Source: CAD feature listing. Evaluate the final solid. Frame: model axes, mm. Face numbers are marked on the shaded views. A direction names the side the tool comes from. Coordinates: 2 decimals unless noted, no trailing zeros. Write each loop counter-clockwise with the first axis right and the second up, starting at its lowest first coordinate (ties: lowest second). Pieces come first, ordered by that corner, then holes. Notation, with made-up numbers: (-29, 18.5) -> (-18, 18.5) arc R8 cw to (-18, 31.5) -> close; hole circle Ø6 at (73.5, -20). An arc over 180 degrees is marked (long way). One line per item, written item: value. Start each with the question number.
1. Line query: line 1 (X direction, y = 5.2, z = 0); line 2 (X direction, y = 3.35, z = 0); line 3 (Y direction, x = 10.5, z = 0). Output: solid intervals per line, ascending.
2. Section query C-C, the plane x = 15. Output: boundary loops of the cut face in (y, z), and give its area (3 significant figures).
3. Section query B-B, the plane x = 10.25. Output: boundary loops of the cut face in (y, z), and give its area (3 significant figures).
4. Mould query, pull axis Y, two halves, no side actions, for the marked faces 1, 2, 3 and 4. Classes: released by +Y, released by -Y, zero draft, split by the parting line, or undercut.
5. Access query for the marked faces 5, 6, 7, 8 and 9. Directions: +Z, -Z, +X, -X, +Y, -Y. A direction counts if a zero-diameter tool reaches every point of the face in a straight line with its end or side. Return the directions, or none.
6. Section query A-A, the plane y = 3. Output: boundary loops of the cut face in (x, z).
7. First-contact query: P1, Ø3, axis at x = 4.5, y = -1.5, coming from the -Z side; P2, Ø3, axis at x = 5, y = 2.5, coming from the +Z side; P3, Ø5, axis at x = 15, z = 0, coming from the +Y side; P4, Ø3.5, axis at y = 0, z = 0, coming from the -X side. Flat tips, straight axial feed; report the tip coordinate or a pass-through.
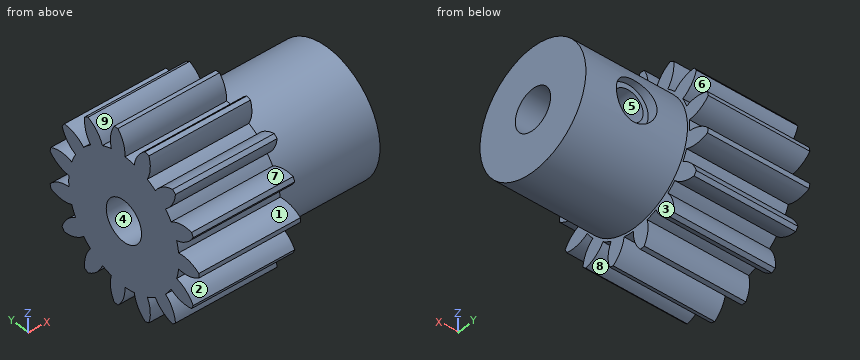
from build123d import *

# Parameters (mm, degrees)
STOCK_GEAR_1M_15T_D4_START_1_OUTLINE_R = 2
STOCK_GEAR_1M_15T_D4_START_1_DEPTH     = 10
SKETCH1_R                              = 6
SKETCH1_R_2                            = 2
BOSS_EXTRUDE1_DEPTH                    = 10
SKETCH2_R                              = 1.5
CUT_EXTRUDE2_DEPTH                     = 6
SKETCH2_3_R                            = 2
CUT_EXTRUDE3_DEPTH                     = 1


# Read off the part's stored shape, not the designer's step: Stock-Gear 1M 15T D4 Start-1
with BuildPart() as part:
    # Stock-Gear 1M 15T D4 Start-1 outline → Stock-Gear 1M 15T D4 Start-1 (new body)
    with BuildSketch(Plane.YZ):
        with BuildLine():
            ThreePointArc((1.106368468, 8.427689411), (0.888491938, 8.453436111), (0.670023493, 8.473551116))
            ThreePointArc((0.670023493, 8.473551116), (0.04560728, 7.441942771), (-0.122166634, 6.24780572))
            ThreePointArc((-0.122166634, 6.24780572), (-0.653198367, 6.214767324), (-1.179494851, 6.136676046))
            ThreePointArc((-1.179494851, 6.136676046), (-1.591877556, 7.26983618), (-2.417132211, 8.149077977))
            ThreePointArc((-2.417132211, 8.149077977), (-2.626644452, 8.083980389), (-2.834406818, 8.013497238))
            ThreePointArc((-2.834406818, 8.013497238), (-2.985246497, 6.817103167), (-2.652816299, 5.657964889))
            ThreePointArc((-2.652816299, 5.657964889), (-3.1245, 5.411792748), (-3.573533178, 5.126388751))
            ThreePointArc((-3.573533178, 5.126388751), (-4.411161274, 5.993850886), (-5.522688773, 6.461416928))
            ThreePointArc((-5.522688773, 6.461416928), (-5.687610154, 6.316731017), (-5.84874244, 6.167836888))
            ThreePointArc((-5.84874244, 6.167836888), (-5.499924035, 5.013524493), (-4.724769925, 4.089810528))
            ThreePointArc((-4.724769925, 4.089810528), (-5.055547198, 3.673070042), (-5.349675154, 3.229702268))
            ThreePointArc((-5.349675154, 3.229702268), (-6.467715133, 3.681474322), (-7.673322273, 3.656518192))
            ThreePointArc((-7.673322273, 3.656518192), (-7.76513639, 3.457261466), (-7.851777359, 3.255701506))
            ThreePointArc((-7.851777359, 3.255701506), (-7.063614741, 2.343061888), (-5.979767908, 1.814490772))
            ThreePointArc((-5.979767908, 1.814490772), (-6.112444357, 1.299240156), (-6.200809696, 0.774570923))
            ThreePointArc((-6.200809696, 0.774570923), (-7.405942289, 0.732537403), (-8.497168643, 0.219374243))
            ThreePointArc((-8.497168643, 0.219374243), (-8.5, 0), (-8.497168643, -0.219374243))
            ThreePointArc((-8.497168643, -0.219374243), (-7.405942289, -0.732537403), (-6.200809696, -0.774570923))
            ThreePointArc((-6.200809696, -0.774570923), (-6.112444357, -1.299240156), (-5.979767908, -1.814490772))
            ThreePointArc((-5.979767908, -1.814490772), (-7.063614741, -2.343061888), (-7.851777359, -3.255701506))
            ThreePointArc((-7.851777359, -3.255701506), (-7.76513639, -3.457261466), (-7.673322273, -3.656518192))
            ThreePointArc((-7.673322273, -3.656518192), (-6.467715133, -3.681474322), (-5.349675154, -3.229702268))
            ThreePointArc((-5.349675154, -3.229702268), (-5.055547198, -3.673070042), (-4.724769925, -4.089810528))
            ThreePointArc((-4.724769925, -4.089810528), (-5.499924035, -5.013524493), (-5.84874244, -6.167836888))
            ThreePointArc((-5.84874244, -6.167836888), (-5.687610154, -6.316731017), (-5.522688773, -6.461416928))
            ThreePointArc((-5.522688773, -6.461416928), (-4.411161274, -5.993850886), (-3.573533178, -5.126388751))
            ThreePointArc((-3.573533178, -5.126388751), (-3.1245, -5.411792748), (-2.652816299, -5.657964889))
            ThreePointArc((-2.652816299, -5.657964889), (-2.985246497, -6.817103167), (-2.834406818, -8.013497238))
            ThreePointArc((-2.834406818, -8.013497238), (-2.626644452, -8.083980389), (-2.417132211, -8.149077977))
            ThreePointArc((-2.417132211, -8.149077977), (-1.591877556, -7.26983618), (-1.179494851, -6.136676046))
            ThreePointArc((-1.179494851, -6.136676046), (-0.653198367, -6.214767324), (-0.122166634, -6.24780572))
            ThreePointArc((-0.122166634, -6.24780572), (0.04560728, -7.441942771), (0.670023493, -8.473551116))
            ThreePointArc((0.670023493, -8.473551116), (0.888491938, -8.453436111), (1.106368468, -8.427689411))
            ThreePointArc((1.106368468, -8.427689411), (1.502656253, -7.288800753), (1.418488851, -6.085876303))
            ThreePointArc((1.418488851, -6.085876303), (1.931047198, -5.94315217), (2.429606752, -5.757344182))
            ThreePointArc((2.429606752, -5.757344182), (3.068575145, -6.780002862), (4.058600654, -7.468451026))
            ThreePointArc((4.058600654, -7.468451026), (4.25, -7.361215932), (4.438567989, -7.249076783))
            ThreePointArc((4.438567989, -7.249076783), (4.337367144, -6.04746546), (3.771202944, -4.982773259))
            ThreePointArc((3.771202944, -4.982773259), (4.181397159, -4.643912014), (4.561279057, -4.271385532))
            ThreePointArc((4.561279057, -4.271385532), (5.560958489, -4.945738865), (6.745408891, -5.171987905))
            ThreePointArc((6.745408891, -5.171987905), (6.876644452, -4.996174644), (7.003298781, -4.817032924))
            ThreePointArc((7.003298781, -4.817032924), (6.422107853, -3.760468449), (5.471841788, -3.018103451))
            ThreePointArc((5.471841788, -3.018103451), (5.708745565, -2.541697283), (5.904264776, -2.046865518))
            ThreePointArc((5.904264776, -2.046865518), (7.091801591, -2.256311686), (8.265874651, -1.981241089))
            ThreePointArc((8.265874651, -1.981241089), (8.314254606, -1.767249372), (8.357095591, -1.55208031))
            ThreePointArc((8.357095591, -1.55208031), (7.396407771, -0.823252281), (6.226349477, -0.531576138))
            ThreePointArc((6.226349477, -0.531576138), (6.249, 0), (6.226349477, 0.531576138))
            ThreePointArc((6.226349477, 0.531576138), (7.396407771, 0.823252281), (8.357095591, 1.55208031))
            ThreePointArc((8.357095591, 1.55208031), (8.314254606, 1.767249372), (8.265874651, 1.981241089))
            ThreePointArc((8.265874651, 1.981241089), (7.091801591, 2.256311686), (5.904264776, 2.046865518))
            ThreePointArc((5.904264776, 2.046865518), (5.708745565, 2.541697283), (5.471841788, 3.018103451))
            ThreePointArc((5.471841788, 3.018103451), (6.422107853, 3.760468449), (7.003298781, 4.817032924))
            ThreePointArc((7.003298781, 4.817032924), (6.876644452, 4.996174644), (6.745408891, 5.171987905))
            ThreePointArc((6.745408891, 5.171987905), (5.560958489, 4.945738865), (4.561279057, 4.271385532))
            ThreePointArc((4.561279057, 4.271385532), (4.181397159, 4.643912014), (3.771202944, 4.982773259))
            ThreePointArc((3.771202944, 4.982773259), (4.337367144, 6.04746546), (4.438567989, 7.249076783))
            ThreePointArc((4.438567989, 7.249076783), (4.25, 7.361215932), (4.058600654, 7.468451026))
            ThreePointArc((4.058600654, 7.468451026), (3.068575145, 6.780002862), (2.429606752, 5.757344182))
            ThreePointArc((2.429606752, 5.757344182), (1.931047198, 5.94315217), (1.418488851, 6.085876303))
            ThreePointArc((1.418488851, 6.085876303), (1.502656253, 7.288800753), (1.106368468, 8.427689411))
        make_face()
        Circle(STOCK_GEAR_1M_15T_D4_START_1_OUTLINE_R, mode=Mode.SUBTRACT)
    extrude(amount=STOCK_GEAR_1M_15T_D4_START_1_DEPTH)

    # Sketch1 → Boss-Extrude1 (add)
    with BuildSketch(Plane(origin=(10, 0, 0), x_dir=(0, 0, -1), z_dir=(1, 0, 0))):
        with Locations(Location((0, 0, 0), (0, 0, 180))):
            Circle(SKETCH1_R)
        Circle(SKETCH1_R_2, mode=Mode.SUBTRACT)
    extrude(amount=BOSS_EXTRUDE1_DEPTH)

    # Sketch2 → Cut-Extrude2 (cut)
    with BuildSketch(Plane(origin=(0, 6, 0), x_dir=(1, 0, 0), z_dir=(0, 1, 0))):
        with Locations(Location((15, 0, 0), (0, 0, 270))):
            Circle(SKETCH2_R)
    extrude(amount=-CUT_EXTRUDE2_DEPTH, mode=Mode.SUBTRACT)

    # Sketch2<3> → Cut-Extrude3 (cut)
    with BuildSketch(Plane(origin=(0, 6, 0), x_dir=(1, 0, 0), z_dir=(0, 1, 0))):
        with Locations(Location((15, 0, 0), (0, 0, 270))):
            Circle(SKETCH2_3_R)
    extrude(amount=-CUT_EXTRUDE3_DEPTH, mode=Mode.SUBTRACT)


solid = part.part
Computed values:
1. line 1: x = 0 to 13, 17 to 20
1. line 2: x = 0 to 13.5, 16.5 to 20
1. line 3: y = -6 to -2, 2 to 6
2. outline: (1.32, -1.5) arc R2 cw (long way) to (1.32, 1.5) -> (5, 1.5) -> (5, 2) -> (5.66, 2) arc R6 ccw (long way) to (5.66, -2) -> (5, -2) -> (5, -1.5) -> close
2. area: 87.4 mm²
3. outline: circle Ø12 at (0, 0); hole circle Ø4 at (0, 0)
3. area: 101 mm²
4. face 1: undercut
4. face 2: released by -Y
4. face 3: zero draft
4. face 4: undercut
5. face 5: +Y
5. face 6: +X, -X, +Y
5. face 7: +X, -X
5. face 8: -Z, +X, -X
5. face 9: +Z, +X, -X
6. outline: (0, -6.71) -> (10, -6.71) -> (10, -5.2) -> (20, -5.2) -> (20, 5.2) -> (10, 5.2) -> (10, 6.71) -> (0, 6.71) -> close; hole circle Ø3 at (15, 0)
7. P1: stops at z = -8.15
7. P2: stops at z = 8.44
7. P3: stops at y = 6
7. P4: passes through
